from build123d import *

# Parameters (mm, degrees)
F3_R      = 125
F4_DEPTH  = 15
F0_R      = 67.5
F6_R      = 117
F7_DEPTH  = 56
F8_W      = 40
F8_H      = 195.041159
F9_DEPTH  = 56
F11_DEPTH = 32


with BuildPart() as f4:
    # F3 (on offset) → F4 (new body)
    with BuildSketch(Plane.YZ.offset(1613)):
        with Locations((0, -350)):
            Circle(F3_R)
    extrude(amount=F4_DEPTH)

    # F5: sweep along a path in F1
    with BuildLine(Plane.XZ) as f5_path:
        Line((0, 0), (0, -150))
        ThreePointArc((0, -150), (58.578644, -291.421356), (200, -350))
        Line((200, -350), (1613, -350))
    # F0 (on Top) → F5 (sweep)
    with BuildSketch(Plane.XY):
        Circle(F0_R)
    sweep(path=f5_path.line)

    # F6 (on offset) → F7 (join)
    with BuildSketch(Plane.YZ.offset(1613)):
        with Locations((0, -351.443887)):
            Circle(F6_R)
    extrude(amount=-F7_DEPTH)

    # F8 (on offset) → F9 (join)
    with BuildSketch(Plane.YZ.offset(1613)):
        with Locations((0, -225.520579)):
            Rectangle(F8_W, F8_H)
    extrude(amount=-F9_DEPTH)

    # F10 (on face) → F11 (join)
    with BuildSketch(Plane.XY.offset(-128)):
        with BuildLine():
            Line((1557, 259.156863), (1557, 20))
            Line((1557, 20), (1613, 20))
            Line((1613, 20), (1613, 259.156863))
            ThreePointArc((1613, 259.156863), (1608.359653, 270.359653), (1597.156863, 275))
            Line((1597.156863, 275), (1572.843137, 275))
            ThreePointArc((1572.843137, 275), (1561.640347, 270.359653), (1557, 259.156863))
        make_face()
    extrude(amount=-F11_DEPTH)


solid = f4.part
Can you work these out from the model? Positions are in its coordinate system, mm. A direction names the side the tool comes from. Coordinates: 2 decimals unless noted, no trailing zeros. Return JSON: item names as keys, results as strings. Group by question number.
Item 1: I'm going to push flat-ended pins straight in: pin 1 Ø4 at (x, y) = (627.5, -28.5) entering from -Z; pin 2 Ø17 at (x, z) = (1576, -184) entering from -Y; pin 3 Ø10 at (y, z) = (28, -113) entering from -X. Where does each tip first touch, or does it pass through?
Item 2: Please list where these lines run through material, in increasing order: probe 1 along Y at (x, z) = (55.5, -287); probe 2 along X at (y, z) = (138, -143); probe 3 along Z at (x, y) = (602.5, -27).
Item 3: We'd pull the mould along Z, two halves only. Please class faces 5 (the face through (1585, 149, -160)), 6 (the face through (1620.395, -27.098, -472.028)), 7 (the face through (1585, -20, -183)): pulls with the +Z half, pulls with the -Z half, needs draft (parallel to the pull), parting line crosses it, or undercut.
Item 4: Which directions (+Z, -Z, +X, -X, +Y, -Y) give clear straight access to the entire face, cutting with the end or side of a thin tool? Please do faces 1 (the face through (-53.57, 41.07, -76.05)), 2 (the face through (1557, 28, -272)), 3 (the face through (1585, 149, -128)), 4 (the face through (1628, -2, -348)).
Return value:
{
 "1": {"pin 1": "stops at z = -412.08", "pin 2": "stops at y = -20", "pin 3": "stops at x = -63.46"},
 "2": {"probe 1": "y = -67.49 to 67.49", "probe 2": "x = 1557 to 1613", "probe 3": "z = -411.86 to -288.14"},
 "3": {"face 5": "undercut", "face 6": "parting line crosses it", "face 7": "needs draft"},
 "4": {"face 1": "+Z", "face 2": "none", "face 3": "+Z, +X, +Y, -Y", "face 4": "+Z, -Z, +X, +Y, -Y"}
}
